Verification items for the finished model (mm, model axes). Face numbers are marked on the shaded views. A direction names the side the tool comes from. Give positions to 0.01 mm unless a question says otherwise; leave off trailing zeros. Order: outer loops, then holes, each group sorted by start corner. A loop starts at its lowest first (then second) coordinate and runs counter-clockwise, first axis right, second up. Notation, with made-up numbers: (-5.5, -8.5) -> (8.5, -8.5) arc R21 ccw to (8.5, 7.5) -> close; hole circle Ø1 at (82.25, 19). An arc over 180 degrees is marked (long way). Return JSON: item names as keys, results as strings. Group by question number.
(1) Tool access check on the marked faces 1, 2 and 3. Record the directions out of +Z, -Z, +X, -X, +Y, -Y that give a thin tool (end or side, any length) a straight path to the whole face; none if there is none.
(2) Depth check by flat-ended pin: pin 1 Ø1.6 at (x, y) = (1, 1) entering from +Z; pin 2 Ø4 at (x, y) = (64, 1) entering from -Z; pin 3 Ø5.5 at (x, y) = (70, 0) entering from -Z; pin 4 Ø5 at (y, z) = (-4.5, 8) entering from +X. Enter the tip coordinate at first touch or a pass-through.
(3) Cross-section at A-A on x = 0. Enter the section's corners in (y, z).
(4) Cross-section at B-B on x = 70. Enter the section's corners in (y, z), then the cut area to 3 significant figures.
(5) Thickness scan on line 1 along X through (y, z) = (0, 1.25); line 2 along X through (y, z) = (0, 1.5); line 3 along Z through (x, y) = (71.5, -0.75). Record the ranges inside material, lowest first.
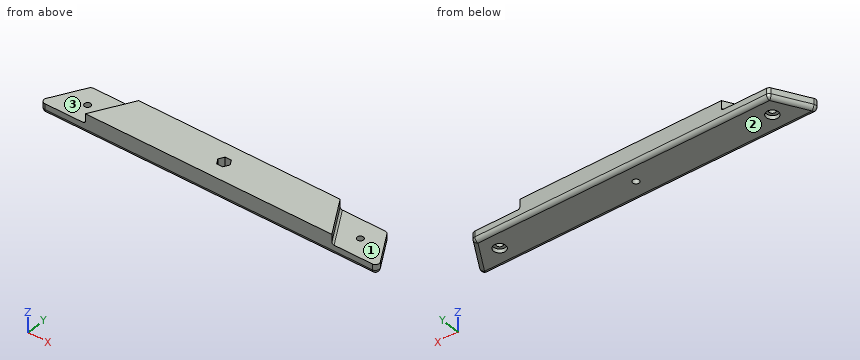
from build123d import *

# Parameters (mm, degrees)
PAD_DEPTH       = 10
POCKET_DEPTH    = 5
SKETCH002_R     = 1.6
POCKET001_DEPTH = 10.001
SKETCH003_R     = 1.6
POCKET002_DEPTH = 362.846575
POCKET003_DEPTH = 5
SKETCH005_R     = 3.1
POCKET004_DEPTH = 2
FILLET_R        = 2
FILLET001_R     = 2
FILLET002_R     = 2
FILLET003_R     = 2
FILLET004_R     = 2
FILLET005_R     = 1
FILLET006_R     = 1


with BuildPart() as part:
    # Sketch → Pad (new body)
    with BuildSketch(Plane.XY):
        Polygon((-75.952995, 10), (-87.5, -10), (87.5, -10), (75.952995, 10), align=None)
    extrude(amount=PAD_DEPTH)

    # Sketch001 → Pocket (cut)
    with BuildSketch(Plane.XY.offset(10)):
        Polygon((-75.952995, 10), (-51.704283, 10), (-63.251289, -10), (-87.5, -10), align=None)
    pocket = extrude(amount=-POCKET_DEPTH, mode=Mode.SUBTRACT)

    # Mirrored: Pocket across Sketch001 V_Axis
    add(pocket.mirror(Plane(origin=(0, 0, 10), x_dir=(0, 0, 1), z_dir=(1, 0, 0))), mode=Mode.SUBTRACT)

    # Sketch002 → Pocket001 (cut, through all)
    with BuildSketch(Plane(origin=(0, 0, 0), x_dir=(1, 0, 0), z_dir=(0, 0, -1))):
        Circle(SKETCH002_R)
    extrude(amount=-POCKET001_DEPTH, mode=Mode.SUBTRACT)

    # Sketch003 → Pocket002 (cut, through all)
    with BuildSketch(Plane(origin=(0, 0, 0), x_dir=(1, 0, 0), z_dir=(0, 0, -1))):
        with Locations((-70, 0)):
            Circle(SKETCH003_R)
    pocket002 = extrude(amount=-POCKET002_DEPTH, mode=Mode.SUBTRACT)

    # Mirrored001: Pocket002 across Sketch003 V_Axis
    add(pocket002.mirror(Plane(origin=(0, 0, 0), x_dir=(0, 0, -1), z_dir=(1, 0, 0))), mode=Mode.SUBTRACT)

    # Sketch004 → Pocket003 (cut)
    with BuildSketch(Plane.XY.offset(10)):
        Polygon((3.175426, 0), (1.587713, 2.75), (-1.587713, 2.75), (-3.175426, 0), (-1.587713, -2.75), (1.587713, -2.75), align=None)
    extrude(amount=-POCKET003_DEPTH, mode=Mode.SUBTRACT)

    # Sketch005 → Pocket004 (cut)
    with BuildSketch(Plane(origin=(0, 0, 0), x_dir=(1, 0, 0), z_dir=(0, 0, -1))):
        with Locations((-70, 0)):
            Circle(SKETCH005_R)
    pocket004 = extrude(amount=-POCKET004_DEPTH, mode=Mode.SUBTRACT)

    # Mirrored002: Pocket004 across Sketch005 V_Axis
    add(pocket004.mirror(Plane(origin=(0, 0, 0), x_dir=(0, 0, -1), z_dir=(1, 0, 0))), mode=Mode.SUBTRACT)

    # Fillet
    fillet_edges = [part.edges().sort_by_distance(p)[0] for p in [
        (-75.952995, 10, 2.5),
    ]]
    fillet(fillet_edges, radius=FILLET_R)

    # Fillet001
    fillet001_edges = [part.edges().sort_by_distance(p)[0] for p in [
        (-87.5, -10, 2.5),
    ]]
    fillet(fillet001_edges, radius=FILLET001_R)

    # Fillet002
    fillet002_edges = [part.edges().sort_by_distance(p)[0] for p in [
        (75.952995, 10, 2.5),
    ]]
    fillet(fillet002_edges, radius=FILLET002_R)

    # Fillet003
    fillet003_edges = [part.edges().sort_by_distance(p)[0] for p in [
        (87.5, -10, 2.5),
    ]]
    fillet(fillet003_edges, radius=FILLET003_R)

    # Fillet004
    fillet004_edges = [part.edges().sort_by_distance(p)[0] for p in [
        (-75.798294, 9.732051, 0),
    ]]
    fillet(fillet004_edges, radius=FILLET004_R)

    # Fillet005
    fillet005_edges = [part.edges().sort_by_distance(p)[0] for p in [
        (57.477786, 0, 5),
    ]]
    fillet(fillet005_edges, radius=FILLET005_R)

    # Fillet006
    fillet006_edges = [part.edges().sort_by_distance(p)[0] for p in [
        (-57.477786, 0, 5),
    ]]
    fillet(fillet006_edges, radius=FILLET006_R)


solid = part.part
Verdict:
{
 "1": {"face 1": "+Z, +X, +Y", "face 2": "-Z, +X, -X, +Y, -Y", "face 3": "+Z, -X, +Y"},
 "2": {"pin 1": "z = 5", "pin 2": "z = 0", "pin 3": "z = 2", "pin 4": "x = 61.52"},
 "3": {"outline": "(-10, 2) arc R2 ccw to (-8, 0) -> (-1.6, 0) -> (-1.6, 5) -> (-2.75, 5) -> (-2.75, 10) -> (-10, 10) -> close; (1.6, 0) -> (8, 0) arc R2 ccw to (10, 2) -> (10, 10) -> (2.75, 10) -> (2.75, 5) -> (1.6, 5) -> close"},
 "4": {"outline": "(-10, 2) arc R2 ccw to (-8, 0) -> (-3.1, 0) -> (-3.1, 2) -> (-1.6, 2) -> (-1.6, 5) -> (-10, 5) -> close; (1.6, 2) -> (3.1, 2) -> (3.1, 0) -> (8, 0) arc R2 ccw to (10, 2) -> (10, 5) -> (1.6, 5) -> close", "area": "76.3 mm²"},
 "5": {"line 1": "-81.56 to -73.1, -66.9 to -1.6, 1.6 to 66.9, 73.1 to 81.56", "line 2": "-81.65 to -73.1, -66.9 to -1.6, 1.6 to 66.9, 73.1 to 81.65", "line 3": "2 to 5"}
}
